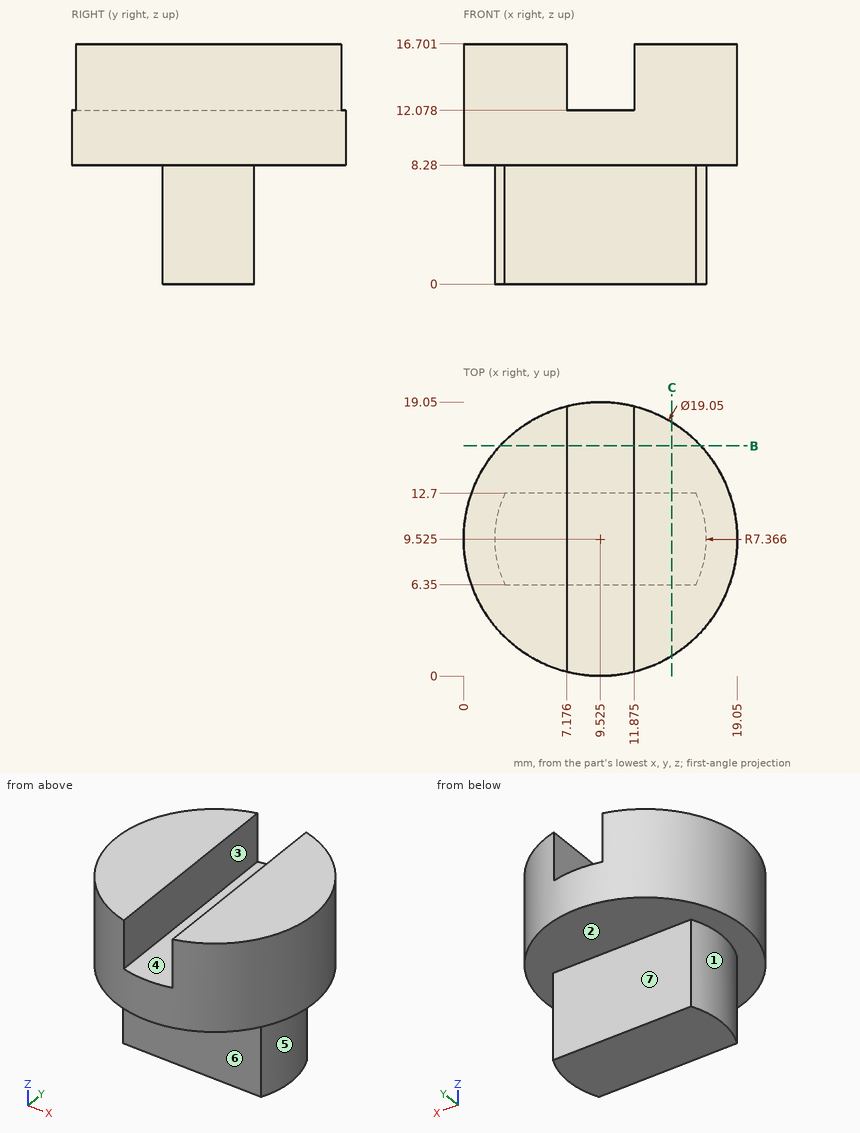
Geometry check sheet. Reference: drawing and pictorial views, mm from the part's lowest x, y, z. A direction names the side the tool comes from. Give positions to 0.01 mm unless a question says otherwise; leave off trailing zeros. Loops run counter-clockwise (first coordinate to the right, second up) from the corner with the lowest first, then second, coordinate; pieces in that order, holes last. Notation, with made-up numbers: (57, 85) - (64, 85) arc R9 ccw to (64, 100) - close; hole circle Ø11 at (4.25, 68.5). An arc over 180 degrees is marked (long way). One line per question, with ' | ' between items. Start each with the question number.
1. Set-up check for the marked faces 4, 5, 6 and 7: record each of +Z, -Z, +X, -X, +Y, -Y from which the full face is reachable in a straight line by a thin tool's end or side.
2. Material ranges on line 1 along Z through (x, y) = (18.25, 12.25); line 2 along Y through (x, z) = (8.5, 3.25); line 3 along Z through (x, y) = (9.25, 15), recorded low to high. Write a range as [from, to].
3. Cross-section at C-C, the plane x = 14.5. Enter the section's corners in (y, z), plus the area to 3 significant figures.
4. Draft check along X on the marked faces 1, 2 and 3. Enter one of: released by +X, released by -X, zero draft, split by the parting line, or undercut.
5. Cross-section at B-B, the plane y = 16. Enter the section's corners in (x, z) (1 decimal).
6. Gauge pin test, flat ends, axial feed: pin 1 Ø4 at (x, z) = (12.5, 3) entering from -Y; pin 2 Ø1.4 at (y, z) = (12, 14) entering from -X; pin 3 Ø2 at (y, z) = (16, 7) entering from -X; pin 4 Ø4 at (x, y) = (12.5, 16) entering from -Z. Record the tip position at first contact, or that the pin passes through.
Check result:
1) face 4: +Z, +Y, -Y | face 5: -Z, +X | face 6: -Z, +X, -X, -Y | face 7: -Z, +X, -X, +Y
2) line 1: z = [8.28, 16.7] | line 2: y = [6.35, 12.7] | line 3: z = [8.28, 12.08]
3) outline: (1.4, 8.28) - (6.35, 8.28) - (6.35, 0) - (12.7, 0) - (12.7, 8.28) - (17.65, 8.28) - (17.65, 16.7) - (1.4, 16.7) - close | area: 189 mm2
4) face 1: released by -X | face 2: zero draft | face 3: undercut
5) outline: (2.5, 8.3) - (16.5, 8.3) - (16.5, 16.7) - (11.9, 16.7) - (11.9, 12.1) - (7.2, 12.1) - (7.2, 16.7) - (2.5, 16.7) - close
6) pin 1: stops at y = 6.35 | pin 2: stops at x = 0.17 | pin 3: passes through | pin 4: stops at z = 8.28
